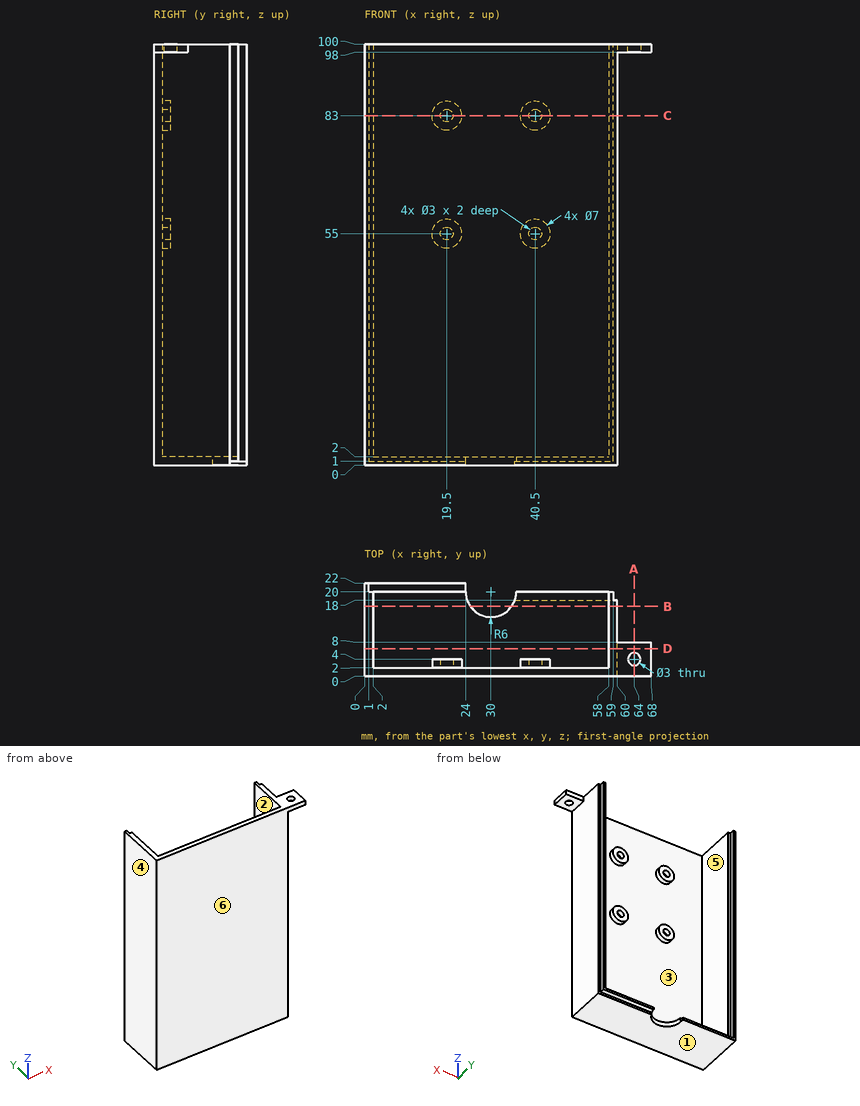
Geometry: see drawing. Coordinates: mm, zero at the bounding-box minimum. A direction names the side the tool comes from. Give positions to 0.01 mm unless a question says otherwise; leave off trailing zeros. Write each loop counter-clockwise with the first axis right and the second up, starting at its lowest first coordinate (ties: lowest second). Pieces come first, ordered by that corner, then holes. Notation, with made-up numbers: (-29.75, 0) - (15.25, 0) arc R18 cw to (15.25, 8) - close; hole circle Ø3 at (46.5, 4). An arc over 180 degrees is marked (long way). Return JSON: item names as keys, results as strings. Group by question number.
1) First-contact query: P1, Ø3.5, axis at x = 39, z = 84.5, coming from the +Y side; P2, Ø1.6, axis at x = 8, y = 20.5, coming from the +Z side; P3, Ø8, axis at x = 57.5, z = 13.5, coming from the +Y side. Flat tips, straight axial feed; report the tip coordinate or a pass-through.
2) Section D-D on y = 6.5. Return the cut outline in (x, z), plus the area to 3 significant figures.
3) Set-up query: the marked faces 1 and 2. Return all of +Z, -Z, +X, -X, +Y, -Y with unobstructed straight access to the full face (end or side cutting, diameter ignored); none if empty.
4) Mould query, pull axis X, two halves, no side actions, for the marked faces 3, 4, 5 and 6. Classes: released by +X, released by -X, zero draft, split by the parting line, or undercut.
5) Line query: line 1 (X direction, y = 2.6, z = 83); line 2 (X direction, y = 8, z = 79); line 3 (Z direction, x = 41, y = 3.5). Output: solid intervals per line, ascending.
6) Section C-C on z = 83. Return the cut outline in (x, y), plus the area to 3 significant figures.
7) Section B-B on y = 16.5. Return the cut outline in (x, z), plus the area to 3 significant figures.
8) Section A-A on x = 64. Return the cut outline in (y, z), plus the area to 3 significant figures.
Filled in:
{
 "1": {"P1": "stops at y = 4", "P2": "stops at z = 2", "P3": "stops at y = 20"},
 "2": {"outline": "(0, 0) - (60, 0) - (60, 98) - (68, 98) - (68, 100) - (58, 100) - (58, 2) - (2, 2) - (2, 100) - (0, 100) - close", "area": "528 mm^2"},
 "3": {"face 1": "-Z, +X, -X, +Y, -Y", "face 2": "+Z, +Y"},
 "4": {"face 3": "undercut", "face 4": "released by -X", "face 5": "undercut", "face 6": "zero draft"},
 "5": {"line 1": "x = 0 to 2, 16 to 18, 21 to 23, 37 to 39, 42 to 44, 58 to 60", "line 2": "x = 0 to 2, 58 to 60", "line 3": "z = 0 to 2, 51.54 to 53.59, 56.41 to 58.46, 79.54 to 81.59, 84.41 to 86.46"},
 "6": {"outline": "(0, 0) - (60, 0) - (60, 18) - (59, 18) - (59, 20) - (58, 20) - (58, 2) - (44, 2) - (44, 4) - (42, 4) - (42, 2) - (39, 2) - (39, 4) - (37, 4) - (37, 2) - (23, 2) - (23, 4) - (21, 4) - (21, 2) - (18, 2) - (18, 4) - (16, 4) - (16, 2) - (2, 2) - (2, 20) - (1, 20) - (1, 22) - (0, 22) - close", "area": "208 mm^2"},
 "7": {"outline": "(0, 0) - (25.13, 0) - (25.13, 2) - (2, 2) - (2, 100) - (0, 100) - close; (34.87, 0) - (60, 0) - (60, 100) - (58, 100) - (58, 2) - (34.87, 2) - close", "area": "493 mm^2"},
 "8": {"outline": "(0, 98) - (2.5, 98) - (2.5, 100) - (0, 100) - close; (5.5, 98) - (8, 98) - (8, 100) - (5.5, 100) - close", "area": "10.0 mm^2"}
}
